Part model, mm, in its own coordinate system. A direction names the side the tool comes from. Round coordinates to 2 decimals unless told otherwise and drop trailing zeros. Loops run counter-clockwise (first coordinate to the right, second up) from the corner with the lowest first, then second, coordinate; pieces in that order, holes last. Notation, with made-up numbers: M 89,60.5 L 142,60.5 A8 cw 142,65.5 Z; hole C -32.75,65 d10. An arc over 180 degrees is marked long. Answer as CSV lines item,"result". Start each with the question number.
Item 1: Wall check: line 1 (Y direction, x = -30.5, z = -6.25); line 2 (X direction, y = 0.45, z = -6.5); line 3 (Z direction, x = -47.5, y = 1.9). Give the ranges that are in metal, low to high.
Item 2: Which spindle directions (+Z, -Z, +X, -X, +Y, -Y) get a long thin tool onto all of the face, cutting with end or side? Do faces 4 (the cylindrical face through (-50.574, 2.699, -8.154)), 5 (the cylindrical face through (-24.16, 1.268, 3.715)), 6 (the cylindrical face through (-41.33, 2.75, -0.1)). Say none if no direction does.
Item 3: Band-saw the part on B-B (z = -5.25). Give the cut face in (x, y), and give its area (3 significant figures).
Item 4: Drop a flat-ended pin along its axis: pin 1 Ø0.8 at (x, y) = (-36, 1) entering from -Z. Give the stop position or say it passes through.
Item 5: Mould opens along Y. For faces 1 (the flat face through (-37, -0.5, -7)), 2 (the flat face through (-49.859, 1, -8)), 3 (the flat face through (-36.9, -0.2, -19)) say: pulls with the +Y half, pulls with the -Y half, needs draft (parallel to the pull), parting line crosses it, or undercut.
Item 6: Band-saw the part on C-C (z = -2). Give the cut face in (x, y), and give its area (3 significant figures).
Item 7: Band-saw the part on A-A (x = -38). Give the cut face in (y, z), and give its area (3 significant figures).
```python
from build123d import *

# Parameters (mm, degrees)
F1_DEPTH = 0.5
F2_DEPTH = 1.25
F5_R     = 1


with BuildPart() as f1:
    # F0 (on Front) → F1 (new body)
    with BuildSketch(Plane.XZ):
        with BuildLine():
            Line((-50.8593195975, 0), (-50.8593195975, -19))
            Line((-50.8593195975, -19), (-49.8593195975, -19))
            Line((-49.8593195975, -19), (-49.8593195975, 3))
            ThreePointArc((-49.8593195975, 3), (-49.5664263787, 3.7071067812), (-48.8593195975, 4))
            Line((-48.8593195975, 4), (-24.8593195975, 4))
            ThreePointArc((-24.8593195975, 4), (-24.1522128163, 3.7071067812), (-23.8593195975, 3))
            Line((-23.8593195975, 3), (-23.8593195975, -19))
            Line((-23.8593195975, -19), (-22.8593195975, -19))
            Line((-22.8593195975, -19), (-22.8593195975, 0))
            Line((-22.8593195975, 0), (-22.8593195975, 3))
            ThreePointArc((-22.8593195975, 3), (-23.4451060351, 4.4142135624), (-24.8593195975, 5))
            Line((-24.8593195975, 5), (-27.8593195975, 5))
            Line((-27.8593195975, 5), (-45.8593195975, 5))
            Line((-45.8593195975, 5), (-48.8593195975, 5))
            ThreePointArc((-48.8593195975, 5), (-50.2735331599, 4.4142135624), (-50.8593195975, 3))
            Line((-50.8593195975, 3), (-50.8593195975, 0))
        make_face()
        with BuildLine():
            Line((-49.8593195975, 3), (-49.8593195975, -19))
            Line((-49.8593195975, -19), (-23.8593195975, -19))
            Line((-23.8593195975, -19), (-23.8593195975, 3))
            ThreePointArc((-23.8593195975, 3), (-24.1522128163, 3.7071067812), (-24.8593195975, 4))
            Line((-24.8593195975, 4), (-48.8593195975, 4))
            ThreePointArc((-48.8593195975, 4), (-49.5664263787, 3.7071067812), (-49.8593195975, 3))
        make_face()
        with BuildLine():
            Line((-41.5405858453, -1.2071067812), (-44.6522128163, -4.3187337522))
            ThreePointArc((-44.6522128163, -4.3187337522), (-45.7420030298, -4.5355065035), (-46.3593195975, -3.611626971))
            Line((-46.3593195975, -3.611626971), (-46.3593195975, -0.5))
            ThreePointArc((-46.3593195975, -0.5), (-46.0664263787, 0.2071067812), (-45.3593195975, 0.5))
            Line((-45.3593195975, 0.5), (-42.2476926265, 0.5))
            ThreePointArc((-42.2476926265, 0.5), (-41.323813094, -0.1173165676), (-41.5405858453, -1.2071067812))
        make_face(mode=Mode.SUBTRACT)
    extrude(amount=F1_DEPTH)

    # F0 (on Front) → F2 (join)
    with BuildSketch(Plane.XZ):
        with BuildLine():
            Line((-50.8593195975, 0), (-50.8593195975, -19))
            Line((-50.8593195975, -19), (-49.8593195975, -19))
            Line((-49.8593195975, -19), (-49.8593195975, 3))
            ThreePointArc((-49.8593195975, 3), (-49.5664263787, 3.7071067812), (-48.8593195975, 4))
            Line((-48.8593195975, 4), (-24.8593195975, 4))
            ThreePointArc((-24.8593195975, 4), (-24.1522128163, 3.7071067812), (-23.8593195975, 3))
            Line((-23.8593195975, 3), (-23.8593195975, -19))
            Line((-23.8593195975, -19), (-22.8593195975, -19))
            Line((-22.8593195975, -19), (-22.8593195975, 0))
            Line((-22.8593195975, 0), (-22.8593195975, 3))
            ThreePointArc((-22.8593195975, 3), (-23.4451060351, 4.4142135624), (-24.8593195975, 5))
            Line((-24.8593195975, 5), (-27.8593195975, 5))
            Line((-27.8593195975, 5), (-45.8593195975, 5))
            Line((-45.8593195975, 5), (-48.8593195975, 5))
            ThreePointArc((-48.8593195975, 5), (-50.2735331599, 4.4142135624), (-50.8593195975, 3))
            Line((-50.8593195975, 3), (-50.8593195975, 0))
        make_face()
    extrude(amount=-F2_DEPTH)

    # F4: F1 across plane


with BuildPart() as f1_1:
    add(f1.part)
    add(f1.part.mirror(Plane(origin=(-36.8593195975, 1.25, -3.0970811102), x_dir=(1, 0, 0), z_dir=(0, 1, 0))))

    # F5
    f5_edges = [f1_1.edges().sort_by_distance(p)[0] for p in [
        (-50.85932, 3, -8),
        (-50.85932, -0.5, -8),
    ]]
    fillet(f5_edges, radius=F5_R)


solid = f1_1.part
```
Answer block:
1,line 1,"y = -0.5 to 0, 2.5 to 3"
1,line 2,"x = -50.86 to -49.86, -23.86 to -22.86"
1,line 3,"z = 4 to 5"
2,face 4,"+Z, -Z, -X, +Y"
2,face 5,"-Z"
2,face 6,"+Y, -Y"
3,outline,"M -50.86,0.5 A1 ccw -49.86,-0.5 L -23.86,-0.5 A1 ccw -22.86,0.5 L -22.86,2 A1 ccw -23.86,3 L -49.86,3 A1 ccw -50.86,2 Z; hole M -49.86,0 L -23.86,0 L -23.86,2.5 L -49.86,2.5 Z"
3,area,"32.1 mm^2"
4,pin 1,"stops at z = 4"
5,face 1,"pulls with the -Y half"
5,face 2,"undercut"
5,face 3,"needs draft"
6,outline,"M -50.86,0.5 A1 ccw -49.86,-0.5 L -46.36,-0.5 L -46.36,0 L -49.86,0 L -49.86,2.5 L -46.36,2.5 L -46.36,3 L -49.86,3 A1 ccw -50.86,2 Z; M -42.33,-0.5 L -23.86,-0.5 A1 ccw -22.86,0.5 L -22.86,2 A1 ccw -23.86,3 L -42.33,3 L -42.33,2.5 L -23.86,2.5 L -23.86,0 L -42.33,0 Z"
6,area,"28.1 mm^2"
7,outline,"M -0.5,-19 L 0,-19 L 0,4 L 2.5,4 L 2.5,-19 L 3,-19 L 3,4 A1 ccw 2,5 L 0.5,5 A1 ccw -0.5,4 Z"
7,area,"26.1 mm^2"
